Could you check a few things on this model? Use its own coordinates, in mm. A direction names the side the tool comes from. Give positions to 0.01 mm unless a question says otherwise; leave off trailing zeros. Loops run counter-clockwise (first coordinate to the right, second up) from the corner with the lowest first, then second, coordinate; pieces in that order, holes last. Notation, with made-up numbers: M -14,22.25 L 21,22.25 A20 ccw 21,60.25 Z; hole C 60,-18 d11. An arc over 180 degrees is marked long. Answer in a Markdown table with one row per item. Add a question column.
1. I'm going to push flat-ended pins straight in: pin 1 Ø1.5 at (x, y) = (4, -21) entering from +Z; pin 2 Ø1 at (x, z) = (48, 6) entering from -Y. Where does each tip first touch, or does it pass through?
2. Thinking about a two-plate mould opening in X: for faces 4 (the flat face through (14, -19, 0)), 5 (the flat face through (48.214, -18, 7)), 6 (the flat face through (45.414, -18, 7)), 7 (the flat face through (47.014, -18, 7)), which applies, released by +X, released by -X, zero draft, split by the parting line, or undercut?
3. If we section it at D-D on z = 1: List the corners of the cut face in (x, y) for me, then the cut area to 3 significant figures.
4. I need wall thicknesses on line 1 along X through (y, z) = (-11, 10.25); line 2 along X through (y, z) = (-16.5, 1.5); line 3 along Y through (x, z) = (9, 4). Which ranges of each line are inside material? Lowest first, please. Write a range as from..to.
5. If we section it at C-C on z = 6: List the corners of the cut face in (x, y) for me, then the cut area to 3 significant figures.
6. If we section it at A-A on x = -11: List the corners of the cut face in (y, z) for me, then the cut area to 3 significant figures.
7. Which directions (+Z, -Z, +X, -X, +Y, -Y) give clear straight access to the entire face, cutting with the end or side of a thin tool? Please do faces 1 (the flat face through (48, -17, 2)), 2 (the cylindrical face through (35.522, -18.343, 0.986)), 3 (the flat face through (12, -9.148, 7)).
8. If we section it at B-B on y = -11.75: List the corners of the cut face in (x, z) for me, then the cut area to 3 significant figures.
```python
from build123d import *

# Parameters (mm, degrees)
F0_W     = 1.5
F0_H     = 16.642398566
F0_W_2   = 1.6
F1_DEPTH = 12
F0_W_3   = 65.7
F0_R     = 1.75
F0_W_4   = 1.2
F2_DEPTH = 2
F3_R     = 3


with BuildPart() as f1:
    # F0 (on Top) → F1 (new body)
    with BuildSketch(Plane.XY):
        Polygon((49.7141629457, -7.7906338274), (-20.2858370543, -7.7906338274), (-20.2858370543, -9.1482352614), (45.4141629457, -9.1482352614), (47.0141629457, -9.1482352614), (48.2141629457, -9.1482352614), (49.7141629457, -9.1482352614), align=None)
        with Locations((48.9641629457, -17.4694345444)):
            Rectangle(F0_W, F0_H)
        with Locations((46.2141629457, -17.4694345444)):
            Rectangle(F0_W_2, F0_H)
    extrude(amount=F1_DEPTH)

    # F0 (on Top) → F2 (join)
    with BuildSketch(Plane.XY):
        with Locations((12.5641629457, -17.4694345444)):
            Rectangle(F0_W_3, F0_H)
        with Locations((-10.2858370543, -16.7906338274)):
            Circle(F0_R, mode=Mode.SUBTRACT)
        with Locations((14.7141629457, -16.7906338274)):
            Circle(F0_R, mode=Mode.SUBTRACT)
        with Locations((34.7141629457, -16.7906338274)):
            Circle(F0_R, mode=Mode.SUBTRACT)
        with Locations((47.6141629457, -17.4694345444)):
            Rectangle(F0_W_4, F0_H)
    extrude(amount=F2_DEPTH)

    # F3
    f3_edges = [f1.edges().sort_by_distance(p)[0] for p in [
        (48.964163, -25.790634, 12),
        (46.214163, -25.790634, 12),
    ]]
    fillet(f3_edges, radius=F3_R)


solid = f1.part
```
Results:
| question | item | result |
|---|---|---|
| 1 | pin 1 | z = 2 |
| 1 | pin 2 | y = -25.79 |
| 2 | face 4 | zero draft |
| 2 | face 5 | undercut |
| 2 | face 6 | released by -X |
| 2 | face 7 | undercut |
| 3 | outline | M -20.29,-25.79 L 49.71,-25.79 L 49.71,-7.79 L -20.29,-7.79 Z; hole C -10.29,-16.79 d3.5; hole C 14.71,-16.79 d3.5; hole C 34.71,-16.79 d3.5 |
| 3 | area | 1,230 mm2 |
| 4 | line 1 | 45.41..47.01, 48.21..49.71 |
| 4 | line 2 | -20.29..-12.01, -8.56..12.99, 16.44..32.99, 36.44..49.71 |
| 4 | line 3 | -9.15..-7.79 |
| 5 | outline | M -20.29,-9.15 L 45.41,-9.15 L 45.41,-25.79 L 47.01,-25.79 L 47.01,-9.15 L 48.21,-9.15 L 48.21,-25.79 L 49.71,-25.79 L 49.71,-7.79 L -20.29,-7.79 Z |
| 5 | area | 147 mm2 |
| 6 | outline | M -25.79,0 L -18.39,0 L -18.39,2 L -25.79,2 Z; M -15.19,0 L -7.79,0 L -7.79,12 L -9.15,12 L -9.15,2 L -15.19,2 Z |
| 6 | area | 43.2 mm2 |
| 7 | face 1 | +Z, -Y |
| 7 | face 2 | +Z, -Z |
| 7 | face 3 | +Z, -X, -Y |
| 8 | outline | M -20.29,0 L 49.71,0 L 49.71,12 L 48.21,12 L 48.21,2 L 47.01,2 L 47.01,12 L 45.41,12 L 45.41,2 L -20.29,2 Z |
| 8 | area | 171 mm2 |
